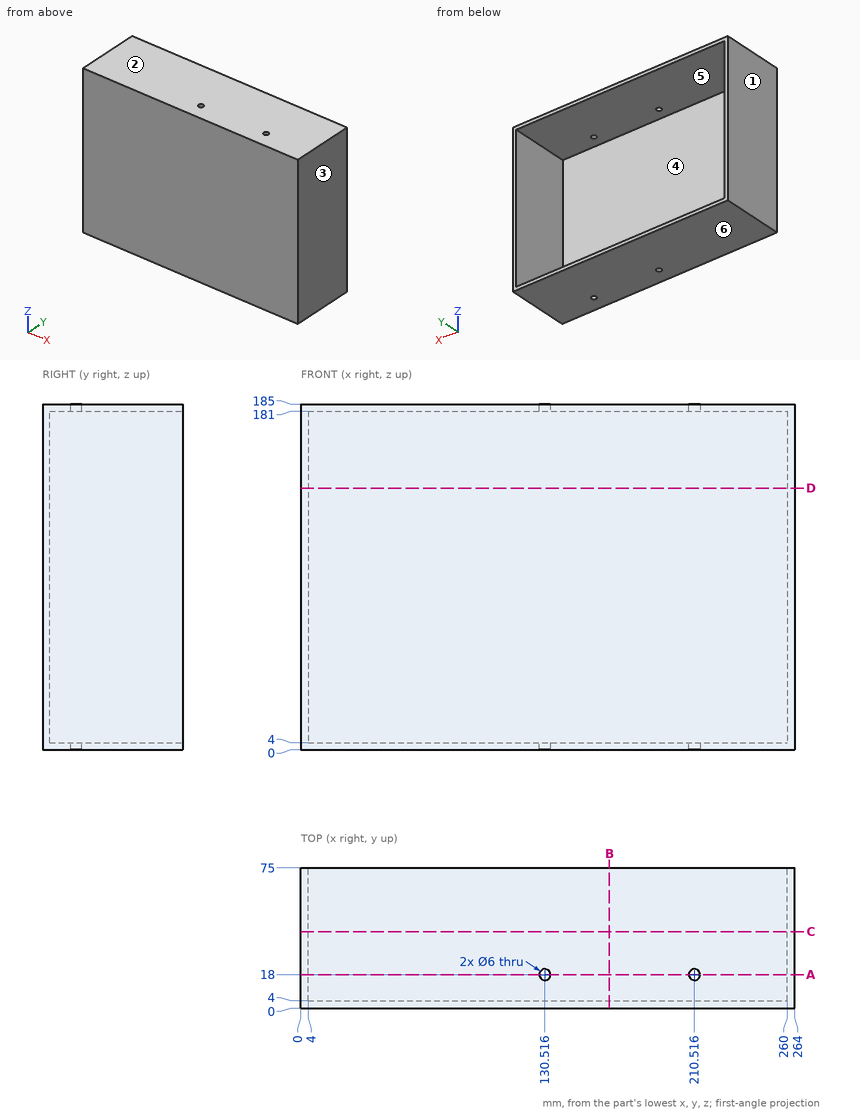
Design review of the part shown in the three views and the two pictorial views. Dimensions are in mm from the part's minimum x, y and z. A direction names the side the tool comes from. Round coordinates to 2 decimals unless told otherwise and drop trailing zeros. Loops run counter-clockwise (first coordinate to the right, second up) from the corner with the lowest first, then second, coordinate; pieces in that order, holes last. Notation, with made-up numbers: (59, 81) - (66, 81) arc R18 ccw to (66, 107) - close; hole circle Ø11 at (26, 51). An arc over 180 degrees is marked (long way). One line per item, written item: value. Start each with the question number.
Item 1: Clearance check with flat-ended pins moving along their axes: pin 1 Ø1 at (x, z) = (223.5, 66.5) entering from +Y; pin 2 Ø5.5 at (x, y) = (210.52, 18) entering from -Z. State where each tip first meets the part, or that it passes through.
Item 2: Take a section at A-A (y = 18). Give the boundary of the cut face in (x, z), plus the area to 3 significant figures.
Item 3: For the marked faces 5 and 6, list the 3-axis set-ups (+Z, -Z, +X, -X, +Y, -Y) from which the entire face can be reached by the end or side of a thin tool; tool diameter is ignored.
Item 4: The part is to be moulded in two halves that separate along X. For the marked faces 1, 2, 3 and 4, say which applies: +X half, -X half, draft (parallel to the pull), parting line (faces both ways), or undercut.
Item 5: For L1, parallel to Z at x = 178, y = 62; L2, parallel to X at y = 8, z = 21.5; L3, parallel to Y at x = 29.5, z = 126, list the stretches that pass through material, from the lowest coordinate up.
Item 6: Take a section at B-B (x = 165). Give the boundary of the cut face in (y, z).
Item 7: Take a section at C-C (y = 41). Give the boundary of the cut face in (x, z).
Item 8: Take a section at D-D (z = 140). Give the boundary of the cut face in (x, y).
Answer below:
1. pin 1: stops at y = 4
1. pin 2: passes through
2. outline: (0, 0) - (127.52, 0) - (127.52, 4) - (4, 4) - (4, 181) - (127.52, 181) - (127.52, 185) - (0, 185) - close; (133.52, 0) - (207.52, 0) - (207.52, 4) - (133.52, 4) - close; (133.52, 181) - (207.52, 181) - (207.52, 185) - (133.52, 185) - close; (213.52, 0) - (264, 0) - (264, 185) - (213.52, 185) - (213.52, 181) - (260, 181) - (260, 4) - (213.52, 4) - close
2. area: 3,430 mm2
3. face 5: +Y
3. face 6: -Z, +X, -X, +Y, -Y
4. face 1: -X half
4. face 2: draft
4. face 3: +X half
4. face 4: undercut
5. L1: z = 0 to 4, 181 to 185
5. L2: x = 0 to 4, 260 to 264
5. L3: y = 0 to 4
6. outline: (0, 0) - (75, 0) - (75, 4) - (4, 4) - (4, 181) - (75, 181) - (75, 185) - (0, 185) - close
7. outline: (0, 0) - (264, 0) - (264, 185) - (0, 185) - close; hole (4, 4) - (260, 4) - (260, 181) - (4, 181) - close
8. outline: (0, 0) - (264, 0) - (264, 75) - (260, 75) - (260, 4) - (4, 4) - (4, 75) - (0, 75) - close
